from build123d import *

# Parameters (mm, degrees)
BOSS_EXTRUDE1_DEPTH = 15.24
BOSS_EXTRUDE2_START = -1.27
BOSS_EXTRUDE2_DEPTH = 1.27
FILLET1_R           = 2.159


with BuildPart() as part:
    # Sketch1 → Boss-Extrude1 (new body)
    with BuildSketch(Plane(origin=(0, 0, 0), x_dir=(1, 0, 0), z_dir=(0, 1, 0))):
        with BuildLine():
            ThreePointArc((-1.27, 27.305), (-0.637643541, 28.831643541), (0.889, 29.464))
            Line((0.889, 29.464), (38.735, 29.464))
            ThreePointArc((38.735, 29.464), (40.261643541, 28.831643541), (40.894, 27.305))
            Line((40.894, 27.305), (40.894, 0.889))
            ThreePointArc((40.894, 0.889), (40.261643541, -0.637643541), (38.735, -1.27))
            Line((38.735, -1.27), (0.889, -1.27))
            ThreePointArc((0.889, -1.27), (-0.637643541, -0.637643541), (-1.27, 0.889))
            Line((-1.27, 0.889), (-1.27, 27.305))
        make_face()
        with BuildLine():
            ThreePointArc((0.889, 28.194), (0.260382072, 27.933617928), (0, 27.305))
            Line((0, 27.305), (0, 0.889))
            ThreePointArc((0, 0.889), (0.260382072, 0.260382072), (0.889, 0))
            Line((0.889, 0), (38.735, 0))
            ThreePointArc((38.735, 0), (39.363617928, 0.260382072), (39.624, 0.889))
            Line((39.624, 0.889), (39.624, 27.305))
            ThreePointArc((39.624, 27.305), (39.363617928, 27.933617928), (38.735, 28.194))
            Line((38.735, 28.194), (0.889, 28.194))
        make_face(mode=Mode.SUBTRACT)
    extrude(amount=BOSS_EXTRUDE1_DEPTH)

    # Sketch2 → Boss-Extrude2 (add)
    with BuildSketch(Plane(origin=(0, 15.24, 0), x_dir=(1, 0, 0), z_dir=(0, 1, 0)).offset(BOSS_EXTRUDE2_START)):
        with BuildLine():
            Line((38.735, 28.194), (0.889, 28.194))
            ThreePointArc((0.889, 28.194), (0.260382072, 27.933617928), (0, 27.305))
            Line((0, 27.305), (0, 0.889))
            ThreePointArc((0, 0.889), (0.260382072, 0.260382072), (0.889, 0))
            Line((0.889, 0), (38.735, 0))
            ThreePointArc((38.735, 0), (39.363617928, 0.260382072), (39.624, 0.889))
            Line((39.624, 0.889), (39.624, 27.305))
            ThreePointArc((39.624, 27.305), (39.363617928, 27.933617928), (38.735, 28.194))
        make_face()
    extrude(amount=BOSS_EXTRUDE2_DEPTH)

    # Fillet1
    fillet1_edges = [part.edges().sort_by_distance(p)[0] for p in [
        (-1.27, 15.24, -14.097),
        (-0.637643541, 15.24, 0.637643541),
        (19.812, 15.24, 1.27),
        (40.261643541, 15.24, 0.637643541),
        (40.894, 15.24, -14.097),
        (40.261643541, 15.24, -28.831643541),
        (19.812, 15.24, -29.464),
        (-0.637643541, 15.24, -28.831643541),
    ]]
    fillet(fillet1_edges, radius=FILLET1_R)


solid = part.part
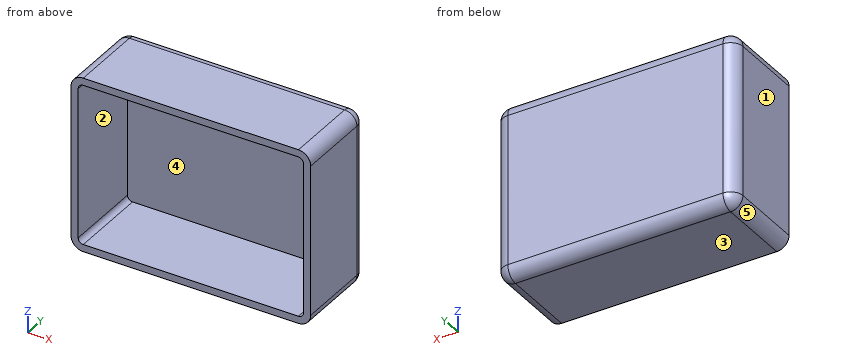
The listing builds one solid part. Answer for the finished solid, in the listing's coordinates (mm). Face numbers are marked on the shaded views. A direction names the side the tool comes from. Coordinates: 2 decimals unless noted, no trailing zeros. Write each loop counter-clockwise with the first axis right and the second up, starting at its lowest first coordinate (ties: lowest second). Pieces come first, ordered by that corner, then holes. Notation, with made-up numbers: M 76.5,48.25 L 95.5,48.25 A20 cw 95.5,66.25 Z; hole C 28,76.25 d6. An arc over 180 degrees is marked long. Use one line per item in the form item = value.
Item 1: Find the intervals of material crossed by probe 1 along Z at (x, y) = (9.5, 11); probe 2 along X at (y, z) = (3.75, -5); probe 3 along Y at (x, z) = (12, -18.5), in increasing order.
Model answer:
probe_1 = -29.46 to -28.19, 0 to 1.27
probe_2 = -1.27 to 0, 39.62 to 40.89
probe_3 = 13.97 to 15.24
Item 2: Find section A-A, the plane y = 1. Give the vertices of the cut face in (x, z) (3 decimals), plus the area to 3 significant figures.
Model answer:
outline = M -1.27,-27.305 A2.159 ccw 0.889,-29.464 L 38.735,-29.464 A2.159 ccw 40.894,-27.305 L 40.894,-0.889 A2.159 ccw 38.735,1.27 L 0.889,1.27 A2.159 ccw -1.27,-0.889 Z; hole M 0,-27.305 A0.889 ccw 0.889,-28.194 L 38.735,-28.194 A0.889 ccw 39.624,-27.305 L 39.624,-0.889 A0.889 ccw 38.735,0 L 0.889,0 A0.889 ccw 0,-0.889 Z
area = 175 mm2
Item 3: Find section B-B, the plane x = 11. Give the vertices of the cut face in (y, z) (3 decimals), plus the area to 3 significant figures.
Model answer:
outline = M 0,-29.464 L 13.081,-29.464 A2.159 ccw 15.24,-27.305 L 15.24,-0.889 A2.159 ccw 13.081,1.27 L 0,1.27 L 0,0 L 13.97,0 L 13.97,-28.194 L 0,-28.194 Z
area = 72.5 mm2
Item 4: Given P1, Ø8.5, axis at x = 26.5, z = -9.5, coming from the -Y side, flat-ended and moving along its own axis, determine where the tip first touches the part or whether it passes through.
Model answer:
P1 = 13.97
Item 5: For the marked faces 4 and 5, determine the directions among +Z, -Z, +X, -X, +Y, -Y from which every point of the face is accessible in a straight line to the end or side of a thin tool.
Model answer:
face_4 = -Y
face_5 = -Z, -X, +Y, -Y
Item 6: Find section C-C, the plane z = -5. Give the vertices of the cut face in (x, y) (3 decimals).
Model answer:
outline = M -1.27,0 L 0,0 L 0,13.97 L 39.624,13.97 L 39.624,0 L 40.894,0 L 40.894,13.081 A2.159 ccw 38.735,15.24 L 0.889,15.24 A2.159 ccw -1.27,13.081 Z
Item 7: The mould has two halves that part along X. Classify the marked faces 1, 2 and 3: released by +X, released by -X, zero draft, split by the parting line, or undercut.
Model answer:
face_1 = released by -X
face_2 = undercut
face_3 = zero draft
